from build123d import *

# Parameters (mm, degrees)
SKETCH_W        = 100
SKETCH_H        = 160
PAD_DEPTH       = 26
SKETCH001_W     = 96
SKETCH001_H     = 156
PAD001_DEPTH    = 28
SKETCH005_W     = 92
SKETCH005_H     = 152
POCKET_DEPTH    = 24
SKETCH003_R     = 9
POCKET001_DEPTH = 28.001
SKETCH002_R     = 1
POCKET002_DEPTH = 28.001
SKETCH006_W     = 96
SKETCH006_H     = 156
POCKET003_DEPTH = 2
SKETCH007_R     = 2.1
POCKET004_DEPTH = 10


with BuildPart() as part:
    # Sketch → Pad (new body)
    with BuildSketch(Plane.XY):
        Rectangle(SKETCH_W, SKETCH_H)
    extrude(amount=PAD_DEPTH)

    # Sketch001 → Pad001 (join)
    with BuildSketch(Plane.XY):
        Rectangle(SKETCH001_W, SKETCH001_H)
    extrude(amount=PAD001_DEPTH)

    # Sketch005 → Pocket (cut)
    with BuildSketch(Plane.XY.offset(28)):
        Rectangle(SKETCH005_W, SKETCH005_H)
    extrude(amount=-POCKET_DEPTH, mode=Mode.SUBTRACT)

    # Sketch003 → Pocket001 (cut, through all)
    with BuildSketch(Plane.XY):
        with Locations((33.25, 36.5)):
            Circle(SKETCH003_R)
        with Locations((25.45, 13.5)):
            Circle(SKETCH003_R)
        with Locations((25.45, -9.5)):
            Circle(SKETCH003_R)
        with Locations((33.25, -32.5)):
            Circle(SKETCH003_R)
        with Locations((-33.25, 36.5)):
            Circle(SKETCH003_R)
        with Locations((-25.45, 13.5)):
            Circle(SKETCH003_R)
        with Locations((-25.45, -9.5)):
            Circle(SKETCH003_R)
        with Locations((-33.25, -32.5)):
            Circle(SKETCH003_R)
    extrude(amount=POCKET001_DEPTH, mode=Mode.SUBTRACT)

    # Sketch002 → Pocket002 (cut, through all)
    with BuildSketch(Plane.XY):
        with Locations((42.25, 72.5)):
            Circle(SKETCH002_R)
        with Locations((-42.25, 72.5)):
            Circle(SKETCH002_R)
        with Locations((42.25, -72.5)):
            Circle(SKETCH002_R)
        with Locations((-42.25, -72.5)):
            Circle(SKETCH002_R)
    extrude(amount=POCKET002_DEPTH, mode=Mode.SUBTRACT)

    # Sketch006 → Pocket003 (cut)
    with BuildSketch(Plane.XY):
        Rectangle(SKETCH006_W, SKETCH006_H)
    extrude(amount=POCKET003_DEPTH, mode=Mode.SUBTRACT)

    # Sketch007 → Pocket004 (cut)
    with BuildSketch(Plane.XZ.offset(80)):
        with Locations((-15, 15)):
            Circle(SKETCH007_R)
        with Locations((-5, 15)):
            Circle(SKETCH007_R)
        with Locations((5, 15)):
            Circle(SKETCH007_R)
        with Locations((15, 15)):
            Circle(SKETCH007_R)
    extrude(amount=-POCKET004_DEPTH, mode=Mode.SUBTRACT)


solid = part.part
Could you check a few things on this model? Use its own coordinates, in mm. A direction names the side the tool comes from. Round coordinates to 2 decimals unless told otherwise and drop trailing zeros. Write each loop counter-clockwise with the first axis right and the second up, starting at its lowest first coordinate (ties: lowest second). Pieces come first, ordered by that corner, then holes. Notation, with made-up numbers: (-0.75, 24) - (26.25, 24) arc R11 ccw to (26.25, 38) - close; hole circle Ø8 at (11, 44). An arc over 180 degrees is marked (long way). Use a Markdown table: item, result.
Q1. Thinking about a two-plate mould opening in Z: for faces 4 (the cylindrical face through (6.13, -78.03, 16.77)), 5 (the cylindrical face through (26.617, 42.583, 2.986)), 6 (the flat face through (-46.4, 0.4, 28)), 7 (the flat face through (-48.4, 0.4, 0)), which applies, released by +Z, released by -Z, zero draft, split by the parting line, or undercut?
Output values:
| item | result |
|---|---|
| face 4 | undercut |
| face 5 | zero draft |
| face 6 | released by +Z |
| face 7 | released by -Z |
Q2. I want a section at D-D (z = 23). List the corners of the cut face in (x, y) for me.
Output values:
| item | result |
|---|---|
| outline | (-50, -80) - (50, -80) - (50, 80) - (-50, 80) - close; hole (-46, -76) - (46, -76) - (46, 76) - (-46, 76) - close |
Q3. I want a section at B-B (x = -5). List the corners of the cut face in (y, z) for me, plus the area to 3 significant figures.
Output values:
| item | result |
|---|---|
| outline | (-80, 0) - (-78, 0) - (-78, 2) - (78, 2) - (78, 0) - (80, 0) - (80, 26) - (78, 26) - (78, 28) - (76, 28) - (76, 4) - (-76, 4) - (-76, 12.9) - (-80, 12.9) - close; (-80, 17.1) - (-76, 17.1) - (-76, 28) - (-78, 28) - (-78, 26) - (-80, 26) - close |
| area | 495 mm2 |
Q4. I want a section at A-A (z = 15). List the corners of the cut face in (x, y) for me.
Output values:
| item | result |
|---|---|
| outline | (-50, -80) - (-17.1, -80) - (-17.1, -76) - (-46, -76) - (-46, 76) - (46, 76) - (46, -76) - (17.1, -76) - (17.1, -80) - (50, -80) - (50, 80) - (-50, 80) - close; (-12.9, -80) - (-7.1, -80) - (-7.1, -76) - (-12.9, -76) - close; (-2.9, -80) - (2.9, -80) - (2.9, -76) - (-2.9, -76) - close; (7.1, -80) - (12.9, -80) - (12.9, -76) - (7.1, -76) - close |
Q5. For faces 1 (the cylindrical face through (16.46, -9.1, 2.99)), 2 (the flat face through (-1, -76, 16)), 3 (the cylindrical face through (-3.87, -78.03, 16.77)), which set-ups out of +Z, -Z, +X, -X, +Y, -Y let a thin tool reach every point of the face, with its end or its side?
Output values:
| item | result |
|---|---|
| face 1 | +Z, -Z |
| face 2 | +Z |
| face 3 | -Y |
Q6. For pin 1 (2.5 mm diameter, centred on x = -42.25, y = -72.5, fed in from +Z); pin 2 (1.6 mm diameter, centred on x = -11.5, z = 27, fed in from -Y); pin 3 (1 mm diameter, centred on x = -8.5, z = 27, fed in from +Y); pin 4 (11 mm diameter, centred on x = 25.45, y = -9.5, fed in from -Z), each with a flat end and sliding along its axis, tell me the tip position at first contact or that it passes through.
Output values:
| item | result |
|---|---|
| pin 1 | z = 4 |
| pin 2 | y = -78 |
| pin 3 | y = 78 |
| pin 4 | through |
Q7. Please list where these lines run through material, in increasing order: L1, parallel to X at y = 13.5, z = 3.1; L2, parallel to X at y = 72.5, z = 2.85; L3, parallel to X at y = -72, z = 24.25.
Output values:
| item | result |
|---|---|
| L1 | -50 to -34.45, -16.45 to 16.45, 34.45 to 50 |
| L2 | -50 to -43.25, -41.25 to 41.25, 43.25 to 50 |
| L3 | -50 to -46, 46 to 50 |
Q8. I want a section at C-C (y = 36.5). List the corners of the cut face in (x, z) for me.
Output values:
| item | result |
|---|---|
| outline | (-50, 0) - (-48, 0) - (-48, 2) - (-42.25, 2) - (-42.25, 4) - (-46, 4) - (-46, 28) - (-48, 28) - (-48, 26) - (-50, 26) - close; (-24.25, 2) - (24.25, 2) - (24.25, 4) - (-24.25, 4) - close; (42.25, 2) - (48, 2) - (48, 0) - (50, 0) - (50, 26) - (48, 26) - (48, 28) - (46, 28) - (46, 4) - (42.25, 4) - close |
